Drawing for the job (mm, zero at the part's lowest x, y, z). A direction names the side the tool comes from. Give positions to 0.01 mm unless a question says otherwise; leave off trailing zeros. Write each loop counter-clockwise with the first axis right and the second up, starting at its lowest first coordinate (ties: lowest second). Pieces come first, ordered by that corner, then holes. Notation, with made-up numbers: (14, 23.5) - (62, 23.5) arc R26 cw to (62, 38.5) - close; hole circle Ø3 at (2, 39). An arc over 180 degrees is marked (long way). Use CSV: the item, a comma, the result in double quotes.
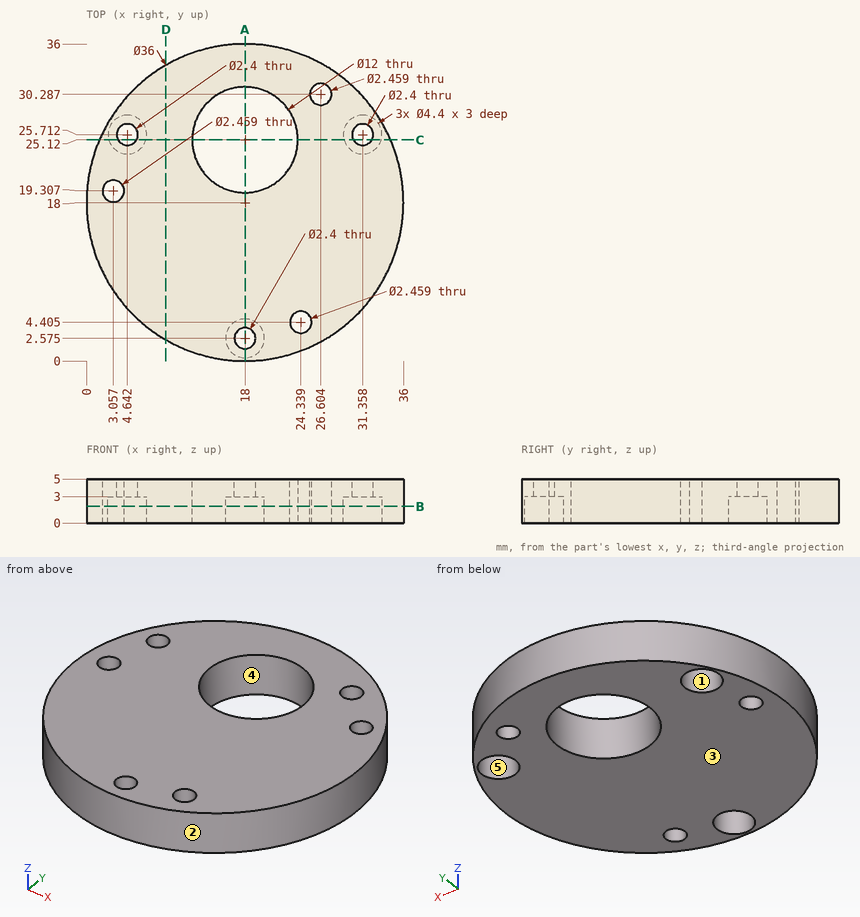
(1) Saw through at B-B, the plane z = 1.9. List the corners of the cut face in (x, y) (1 decimal).
Checked values:
outline,"circle Ø36 at (18, 18); hole circle Ø2.5 at (3.1, 19.3); hole circle Ø4.4 at (4.6, 25.7); hole circle Ø12 at (18, 25.1); hole circle Ø4.4 at (18, 2.6); hole circle Ø2.5 at (24.3, 4.4); hole circle Ø2.5 at (26.6, 30.3); hole circle Ø4.4 at (31.4, 25.7)"
(2) Saw through at D-D, the plane x = 9. List the corners of the cut face in (y, z), then the cut area to 3 significant figures.
Checked values:
outline,"(2.41, 0) - (33.59, 0) - (33.59, 5) - (2.41, 5) - close"
area,"156 mm^2"
(3) Saw through at A-A, the plane x = 18. Count the separate pieces of the cut face and the enclosed holes in it, then the cut area to 3 significant figures.
Checked values:
separate pieces,"3"
enclosed holes,"0"
area,"102 mm^2"
(4) Saw through at C-C, the plane y = 25.12. List the corners of the cut face in (x, z) (1 decimal).
Checked values:
outline,"(1.5, 0) - (2.5, 0) - (2.5, 3) - (3.6, 3) - (3.6, 5) - (1.5, 5) - close; (5.7, 3) - (6.8, 3) - (6.8, 0) - (12, 0) - (12, 5) - (5.7, 5) - close; (24, 0) - (29.2, 0) - (29.2, 3) - (30.3, 3) - (30.3, 5) - (24, 5) - close; (32.4, 3) - (33.5, 3) - (33.5, 0) - (34.5, 0) - (34.5, 5) - (32.4, 5) - close"
(5) Flat gauge pins, fed straight in: P1, Ø2, axis at y = 27.5, z = 3.5, coming from the -X side; P2, Ø1.5, axis at x = 31.5, z = 1, coming from the -Y side (1 decimal); P3, Ø1.3, axis at x = 17.5, y = 3.5, coming from the -Z side. Where does each tip first touch, or does it go through?
Checked values:
P1,"stops at x = 2.13"
P2,"stops at y = 5.3"
P3,"stops at z = 3"
(6) Pull direction Y, two halves, no side cores. Call the marked faces 1, 2 and 3: released by +Y, released by -Y, zero draft, split by the parting line, or undercut.
Checked values:
face 1,"undercut"
face 2,"split by the parting line"
face 3,"zero draft"
(7) 3-axis set-ups, long thin cutter, end or side, ignore diameter. For the marked faces 4 and 5: which of +Z, -Z, +X, -X, +Y, -Y reach the whole face in a straight line?
Checked values:
face 4,"+Z, -Z"
face 5,"-Z"
(8) Wall check: probe 1 along Y at (x, z) = (18, 3.75) (1 decimal); probe 2 along X at (y, z) = (4.5, 2.4) (1 decimal); probe 3 along Y at (x, z) = (27.5, 3.2) (1 decimal). Give the ranges that are in metal, low to high. Write a range as [from, to].
Checked values:
probe 1,"y = [0, 1.4], [3.8, 19.1], [31.1, 36]"
probe 2,"x = [6.1, 16.9], [19.1, 23.1], [25.6, 29.9]"
probe 3,"y = [2.7, 29.4], [31.1, 33.3]"
